CAD build for the part. Positions are in the model's coordinates, mm. Face numbers are marked on the shaded views. Give positions to 0.01 mm unless a question says otherwise; leave off trailing zeros. Write each loop counter-clockwise with the first axis right and the second up, starting at its lowest first coordinate (ties: lowest second). Pieces come first, ordered by that corner, then holes. Notation, with made-up numbers: (-18.75, -3.75) -> (5.25, -3.75) arc R19 ccw to (5.25, 25.25) -> close; hole circle Ø1 at (-15, 31). An arc over 180 degrees is marked (long way). Answer as a JSON object with one key per item and string values.
```python
from build123d import *

# Parameters (mm, degrees)
BOSS_EXTRUDE1_DEPTH     = 12.065
SKETCH6_R               = 9.525
BOSS_EXTRUDE2_DEPTH     = 15.25
CUT_EXTRUDE2_START      = -15.25
SKETCH6_7_R             = 9.525
CUT_EXTRUDE2_DEPTH      = 15.25
CUT_EXTRUDE2_DRAFT      = 3
MIRROR2_START           = -15.25
MIRROR2_COPY_1_SKETCH_R = 9.525
MIRROR2_COPY_1_DEPTH    = 15.25
MIRROR2_COPY_1_DRAFT    = 3


with BuildPart() as part:
    # Sketch2 → Boss-Extrude1 (new, symmetric)
    with BuildSketch(Plane(origin=(0, 0, 0), x_dir=(0, 0, -1), z_dir=(1, 0, 0))):
        with BuildLine():
            Line((-50.8, 0), (-38.1, 0))
            ThreePointArc((-38.1, 0), (0, 38.1), (38.1, 0))
            Line((38.1, 0), (50.8, 0))
            ThreePointArc((50.8, 0), (0, 50.8), (-50.8, 0))
        make_face()
    extrude(amount=BOSS_EXTRUDE1_DEPTH, both=True)

    # Sketch6 → Boss-Extrude2 (add)
    with BuildSketch(Plane.XZ):
        with Locations((0, -50.8)):
            Circle(SKETCH6_R)
    boss_extrude2 = extrude(amount=-BOSS_EXTRUDE2_DEPTH)


with BuildPart() as cut_extrude2_tool:
    # Sketch6<7> → Cut-Extrude2 (with draft: the straight prism first)
    with BuildSketch(Plane.XZ.offset(CUT_EXTRUDE2_START)):
        with Locations((0, -50.8)):
            Circle(SKETCH6_7_R)
    extrude(amount=-CUT_EXTRUDE2_DEPTH)
    # Cut-Extrude2: the draft: its side faces are tilted about the plane it starts from
    cut_extrude2_sides = [cut_extrude2_tool.faces().sort_by_distance(p)[0] for p in [
        (-9.525, 22.875, -50.8),
    ]]
    draft(cut_extrude2_sides, Plane.XZ.offset(CUT_EXTRUDE2_START), CUT_EXTRUDE2_DRAFT)


with BuildPart() as part_1:
    add(part.part)

    # Cut-Extrude2: cut by cut_extrude2_tool
    add(cut_extrude2_tool.part, mode=Mode.SUBTRACT)

    # Sketch15 → CBORE for 5/16 Socket Head Cap Screw1 (revolve, cut)
    with BuildSketch(Plane(origin=(0, 15.25, -50.8), x_dir=(0, 0, 1), z_dir=(1, 0, 0))):
        Polygon((0, 0), (0, 15.25), (4.2164, 15.25), (4.2164, 7.9375), (6.74751, 7.9375), (6.74751, 0.635), (7.38251, 0), align=None)
    cbore_for_5_16_socket_head_cap_screw1 = revolve(axis=Axis((0, 21.6, -50.8), (0, -1, 0)), mode=Mode.SUBTRACT)

    # Mirror2: Boss-Extrude2, CBORE for 5/16 Socket Head Cap Screw1 across plane
    add(boss_extrude2.mirror(Plane.XY))
    add(cbore_for_5_16_socket_head_cap_screw1.mirror(Plane.XY), mode=Mode.SUBTRACT)


with BuildPart() as mirror2_copy_1_tool:
    # Mirror2 copy 1 sketch → Mirror2 copy 1 (with draft: the straight prism first)
    with BuildSketch(Plane.XZ.offset(MIRROR2_START)):
        with Locations((0, 50.8)):
            Circle(MIRROR2_COPY_1_SKETCH_R)
    extrude(amount=-MIRROR2_COPY_1_DEPTH)
    # Mirror2 copy 1: the draft: its side faces are tilted about the plane it starts from
    mirror2_copy_1_sides = [mirror2_copy_1_tool.faces().sort_by_distance(p)[0] for p in [
        (-9.525, 22.875, 50.8),
    ]]
    draft(mirror2_copy_1_sides, Plane.XZ.offset(MIRROR2_START), MIRROR2_COPY_1_DRAFT)


with BuildPart() as part_2:
    add(part_1.part)

    # Mirror2 copy 1: cut by mirror2_copy_1_tool
    add(mirror2_copy_1_tool.part, mode=Mode.SUBTRACT)


solid = part_2.part
```
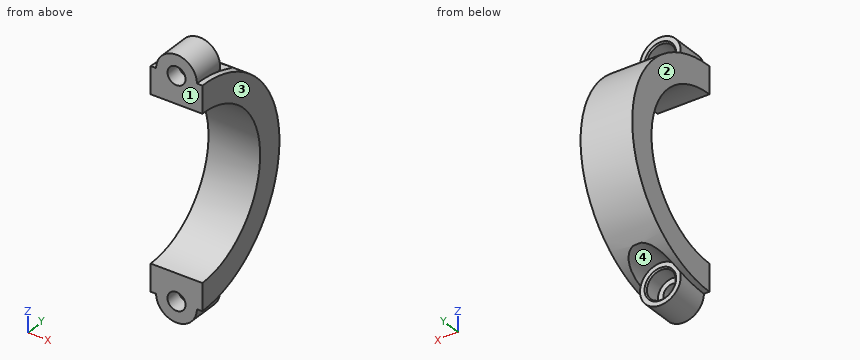
1) Slice it at B-B (z = 0). List the corners of the cut face in (x, y) (3 decimals).
Model answer:
{"outline": "(-12.065, 38.1) -> (12.065, 38.1) -> (12.065, 50.8) -> (-12.065, 50.8) -> close"}
2) Slice it at A-A (x = 0). State how many separate pieces and enclosed holes the cut face has, then the cut area to 3 significant figures.
Model answer:
{"separate pieces": "3", "enclosed holes": "0", "area": "1,620 mm2"}
3) Wall check: probe 1 along X at (y, z) = (11.5, -50.8) (3 decimals); probe 2 along Z at (x, y) = (3.5, 14); probe 3 along Z at (x, y) = (0, 10.25) (1 decimal). Give the ranges that are in metal, low to high.
Model answer:
{"probe 1": "x = -9.525 to -6.748, 6.748 to 9.525", "probe 2": "z = -59.66 to -56.57, -45.03 to -35.43, 35.43 to 45.03, 56.57 to 59.66", "probe 3": "z = -60.3 to -57.5, -44.1 to -36.7, 36.7 to 44.1, 57.5 to 60.3"}
4) Mould opens along X. For the marked faces 1, 2, 3 and 4 say: released by +X, released by -X, zero draft, split by the parting line, or undercut.
Model answer:
{"face 1": "zero draft", "face 2": "released by -X", "face 3": "released by +X", "face 4": "undercut"}
5) Pin check, flat tips, straight feed: pin 1 (8 mm diameter, centred on x = -9.5, y = 8, fed in from +Z); pin 2 (11 mm diameter, centred on x = 0, z = 50.8, fed in from +Y); pin 3 (9.5 mm diameter, centred on x = 4.5, z = 46.5, fed in from +Y). Stop position of each tip, or through.
Model answer:
{"pin 1": "stops at z = 58.58", "pin 2": "stops at y = 7.31", "pin 3": "stops at y = 28.93"}
6) Slice it at C-C (z = -33). List the corners of the cut face in (x, y) (3 decimals), then the cut area to 3 significant figures.
Model answer:
{"outline": "(-12.065, 19.042) -> (12.065, 19.042) -> (12.065, 38.622) -> (-12.065, 38.622) -> close", "area": "472 mm2"}
